from build123d import *

# Parameters (mm, degrees)
SKETCH1_W            = 133
SKETCH1_H            = 133
BOSS_EXTRUDE2_DEPTH  = 136
SKETCH2_W            = 133
SKETCH2_H            = 118
CUT_EXTRUDE1_DEPTH   = 136
BOSS_EXTRUDE3_DEPTH  = 10.5
SKETCH5_W            = 21
SKETCH5_H            = 3
BOSS_EXTRUDE4_DEPTH  = 23.5
SKETCH6_W            = 42
SKETCH6_H            = 17.2
CUT_EXTRUDE2_DEPTH   = 3
BOSS_EXTRUDE5_DEPTH  = 10.5
SKETCH8_W            = 21
SKETCH8_H            = 3
BOSS_EXTRUDE6_DEPTH  = 23.5
SKETCH9_W            = 42
SKETCH9_H            = 17.2
CUT_EXTRUDE3_DEPTH   = 3
SKETCH10_W           = 19.261488562
SKETCH10_H           = 133
BOSS_EXTRUDE7_DEPTH  = 5
SKETCH11_W           = 18.43727499
SKETCH11_H           = 133
BOSS_EXTRUDE8_DEPTH  = 5
SKETCH12_W           = 18.849381776
SKETCH12_H           = 146
BOSS_EXTRUDE9_DEPTH  = 12
SKETCH14_W           = 18.849381776
SKETCH14_H           = 146
BOSS_EXTRUDE10_DEPTH = 12
SKETCH17_R           = 1
CUT_EXTRUDE4_DEPTH   = 222.251553667
SKETCH18_W           = 133
SKETCH18_H           = 136
CUT_EXTRUDE5_DEPTH   = 170
SKETCH20_R           = 2.5
CUT_EXTRUDE6_DEPTH   = 10
SKETCH22_R           = 2.5
CUT_EXTRUDE8_DEPTH   = 170
SKETCH24_R           = 2.5
CUT_EXTRUDE9_DEPTH   = 170
SKETCH26_R           = 2.474722671
CUT_EXTRUDE10_DEPTH  = 177
SKETCH27_R           = 2.5
CUT_EXTRUDE11_DEPTH  = 177
SKETCH29_R           = 2.5
CUT_EXTRUDE12_DEPTH  = 177
SKETCH31_R           = 4
CUT_EXTRUDE13_DEPTH  = 173


with BuildPart() as part:
    # Sketch1 → Boss-Extrude2 (new body)
    with BuildSketch(Plane(origin=(0, 0, 0), x_dir=(1, 0, 0), z_dir=(0, 1, 0))):
        Rectangle(SKETCH1_W, SKETCH1_H)
    extrude(amount=BOSS_EXTRUDE2_DEPTH)

    # Sketch2 → Cut-Extrude1 (cut)
    with BuildSketch(Plane.XY.offset(66.5)):
        with Locations((0, 68)):
            Rectangle(SKETCH2_W, SKETCH2_H)
    extrude(amount=-CUT_EXTRUDE1_DEPTH, mode=Mode.SUBTRACT)


with BuildPart() as cut_extrude1_piece_1:
    # of the separate pieces the step leaves, piece 1, a body of its own (cut_extrude1_pieces)
    add(part.part.solids().sort_by_distance((-66.5, 0, 66.5))[0])

    # Sketch4 → Boss-Extrude3 (add)
    with BuildSketch(Plane(origin=(0, 9, 0), x_dir=(1, 0, 0), z_dir=(0, 1, 0))):
        Polygon((22.75, -22.75), (43.75, -22.75), (46.25, -22.75), (46.25, -20.25), (20.25, -20.25), (20.25, -46.25), (46.25, -46.25), (46.25, -43.75), (43.75, -43.75), (22.75, -43.75), align=None)
        Polygon((22.75, 43.75), (43.75, 43.75), (46.25, 43.75), (46.25, 46.25), (20.25, 46.25), (20.25, 20.25), (46.25, 20.25), (46.25, 22.75), (43.75, 22.75), (22.75, 22.75), align=None)
    extrude(amount=BOSS_EXTRUDE3_DEPTH)

    # Sketch5 → Boss-Extrude4 (add)
    with BuildSketch(Plane(origin=(22.75, 0, 0), x_dir=(0, 0, -1), z_dir=(1, 0, 0))):
        with Locations((-33.25, 18)):
            Rectangle(SKETCH5_W, SKETCH5_H)
        with Locations((33.25, 18)):
            Rectangle(SKETCH5_W, SKETCH5_H)
    extrude(amount=BOSS_EXTRUDE4_DEPTH)

    # Sketch6 → Cut-Extrude2 (cut)
    with BuildSketch(Plane(origin=(0, 19.5, 0), x_dir=(1, 0, 0), z_dir=(0, 1, 0))):
        with Locations((46.25, -33.25)):
            Rectangle(SKETCH6_W, SKETCH6_H)
        with Locations((46.25, 33.25)):
            Rectangle(SKETCH6_W, SKETCH6_H)
    extrude(amount=-CUT_EXTRUDE2_DEPTH, mode=Mode.SUBTRACT)

    # Sketch10 → Boss-Extrude7 (add)
    with BuildSketch(Plane.XZ):
        Rectangle(SKETCH10_W, SKETCH10_H)
    extrude(amount=BOSS_EXTRUDE7_DEPTH)



with BuildPart() as cut_extrude1_piece_2:
    # of the separate pieces the step leaves, piece 2, a body of its own (cut_extrude1_pieces)
    add(part.part.solids().sort_by_distance((66.5, 127, 66.5))[0])

    # Sketch7 → Boss-Extrude5 (add)
    with BuildSketch(Plane.XZ.offset(-127)):
        Polygon((-43.75, 43.75), (-22.75, 43.75), (-22.75, 22.75), (-43.75, 22.75), (-46.25, 22.75), (-46.25, 20.25), (-20.25, 20.25), (-20.25, 46.25), (-46.25, 46.25), (-46.25, 43.75), align=None)
        Polygon((-43.75, -22.75), (-22.75, -22.75), (-22.75, -43.75), (-43.75, -43.75), (-46.25, -43.75), (-46.25, -46.25), (-20.25, -46.25), (-20.25, -20.25), (-46.25, -20.25), (-46.25, -22.75), align=None)
    extrude(amount=BOSS_EXTRUDE5_DEPTH)

    # Sketch8 → Boss-Extrude6 (add)
    with BuildSketch(Plane.ZY.offset(22.75)):
        with Locations((33.25, 118)):
            Rectangle(SKETCH8_W, SKETCH8_H)
        with Locations((-33.25, 118)):
            Rectangle(SKETCH8_W, SKETCH8_H)
    extrude(amount=BOSS_EXTRUDE6_DEPTH)

    # Sketch9 → Cut-Extrude3 (cut)
    with BuildSketch(Plane.XZ.offset(-116.5)):
        with Locations((-46.25, 33.25)):
            Rectangle(SKETCH9_W, SKETCH9_H)
        with Locations((-46.25, -33.25)):
            Rectangle(SKETCH9_W, SKETCH9_H)
    extrude(amount=-CUT_EXTRUDE3_DEPTH, mode=Mode.SUBTRACT)

    # Sketch11 → Boss-Extrude8 (add)
    with BuildSketch(Plane(origin=(0, 136, 0), x_dir=(1, 0, 0), z_dir=(0, 1, 0))):
        Rectangle(SKETCH11_W, SKETCH11_H)
    extrude(amount=BOSS_EXTRUDE8_DEPTH)


with BuildPart() as cut_extrude1_piece_1_1:
    add(cut_extrude1_piece_1.part)

    add(cut_extrude1_piece_2.part)  # Boss-Extrude9 merges Cut-Extrude1 piece 2
    # Sketch12 → Boss-Extrude9 (add)
    with BuildSketch(Plane(origin=(0, 0, -66.5), x_dir=(-1, 0, 0), z_dir=(0, 0, -1))):
        with Locations((-0.206053393, 68)):
            Rectangle(SKETCH12_W, SKETCH12_H)
    extrude(amount=BOSS_EXTRUDE9_DEPTH)

    # Sketch14 → Boss-Extrude10 (add)
    with BuildSketch(Plane.XY.offset(66.5)):
        with Locations((0.206053393, 68)):
            Rectangle(SKETCH14_W, SKETCH14_H)
    extrude(amount=BOSS_EXTRUDE10_DEPTH)

    # Sketch17 → Cut-Extrude4 (cut, through all)
    with BuildSketch(Plane.XY.offset(78.5)):
        with Locations((0.206053393, 68)):
            Circle(SKETCH17_R)
    extrude(amount=-CUT_EXTRUDE4_DEPTH, mode=Mode.SUBTRACT)

    # Sketch18 → Cut-Extrude5 (cut)
    with BuildSketch(Plane.ZY.offset(66.5)):
        with Locations((0, 68)):
            Rectangle(SKETCH18_W, SKETCH18_H)
    extrude(amount=-CUT_EXTRUDE5_DEPTH, mode=Mode.SUBTRACT)

    # Sketch20 → Cut-Extrude6 (cut)
    with BuildSketch(Plane(origin=(0, 0, 0), x_dir=(1, 0, 0), z_dir=(0, 1, 0))):
        with Locations(Location((0, 0, 0), (0, 0, 270))):
            Circle(SKETCH20_R)
    extrude(amount=-CUT_EXTRUDE6_DEPTH, mode=Mode.SUBTRACT)

    # Sketch22 → Cut-Extrude8 (cut)
    with BuildSketch(Plane(origin=(0, 0, 0), x_dir=(1, 0, 0), z_dir=(0, 1, 0))):
        with Locations(Location((0, 0, 0), (0, 0, 270))):
            Circle(SKETCH22_R)
    extrude(amount=CUT_EXTRUDE8_DEPTH, mode=Mode.SUBTRACT)

    # Sketch24 → Cut-Extrude9 (cut)
    with BuildSketch(Plane(origin=(0, 0, 0), x_dir=(1, 0, 0), z_dir=(0, 1, 0))):
        with Locations(Location((0, 59.159797643, 0), (0, 0, 270))):
            Circle(SKETCH24_R)
    extrude(amount=-CUT_EXTRUDE9_DEPTH, mode=Mode.SUBTRACT)

    # Sketch26 → Cut-Extrude10 (cut)
    with BuildSketch(Plane(origin=(0, 9, 0), x_dir=(1, 0, 0), z_dir=(0, 1, 0))):
        with Locations(Location((0, 59.159797643, 0), (0, 0, 90))):
            Circle(SKETCH26_R)
    extrude(amount=CUT_EXTRUDE10_DEPTH, mode=Mode.SUBTRACT)

    # Sketch27 → Cut-Extrude11 (cut)
    with BuildSketch(Plane(origin=(0, 0, 0), x_dir=(1, 0, 0), z_dir=(0, 1, 0))):
        with Locations(Location((0, -59.499471122, 0), (0, 0, 270))):
            Circle(SKETCH27_R)
    extrude(amount=-CUT_EXTRUDE11_DEPTH, mode=Mode.SUBTRACT)

    # Sketch29 → Cut-Extrude12 (cut)
    with BuildSketch(Plane.XZ.offset(5)):
        with Locations(Location((0, 59.499471122, 0), (0, 0, 90))):
            Circle(SKETCH29_R)
    extrude(amount=-CUT_EXTRUDE12_DEPTH, mode=Mode.SUBTRACT)

    # Sketch31 → Cut-Extrude13 (cut)
    with BuildSketch(Plane(origin=(0, 141, 0), x_dir=(1, 0, 0), z_dir=(0, 1, 0))):
        with Locations(Location((0, 0, 0), (0, 0, 270))):
            Circle(SKETCH31_R)
    extrude(amount=-CUT_EXTRUDE13_DEPTH, mode=Mode.SUBTRACT)


solid = cut_extrude1_piece_1_1.part
The listing builds one solid part. Answer for the finished solid, in the listing's coordinates (mm). A direction names the side the tool comes from. Coordinates: 2 decimals unless noted, no trailing zeros. Order: outer loops, then holes, each group sorted by start corner. A loop starts at its lowest first (then second) coordinate and runs counter-clockwise, first axis right, second up. Notation, with made-up numbers: (45, 12) -> (68, 12) arc R24 cw to (68, 33) -> close; hole circle Ø3 at (70.25, 22.25). An arc over 180 degrees is marked (long way). Answer in a Markdown table with one row per item. Add a question column.
Item 1: Which of the six approach directions +Z, -Z, +X, -X, +Y, -Y give full straight-line access (tool end or side, diameter ignored) to faces 5 (the face through (-4.4, -5, -1.1)), 6 (the face through (9.219, 138, 1)), 7 (the face through (-4.2, 136, -0.9))?
Item 2: Find section A-A (z = 0). Write down the section's boundary in (x, y).
Item 3: Determine the mould class of faces 1 (the face through (0, -2, 57)), 2 (the face through (9.631, -3, 0)), 3 (the face through (0.11, -2.465, -61.657)), 4 (the face through (-2, 69, 78.5)) for opening direction Z: +Z half, -Z half, draft (parallel to the pull), parting line (faces both ways), or undercut.
Item 4: Find section C-C (z = 32.5). Write down the section's boundary in (x, y).
Item 5: Find section B-B (y = 13). Write down the section's boundary in (x, z), then the cut area to 3 significant figures.
Item 6: Each of these flat-tipped pins is pushed along its axis until it touches: P1, Ø0.5, axis at x = -9.5, y = -2.5, coming from the -Z side; P2, Ø1.5, axis at y = 139, z = 6, coming from the +X side. Where does it stop, or does it pass through?
Item 7: Find the intervals of material crossed by L1, parallel to Y at x = 4, z = -59.5; L2, parallel to X at y = -3.9, z = 0; L3, parallel to Z at x = 8.25, y = 18, in increasing order. Write a range as from..to.
Result set:
| question | item | result |
|---|---|---|
| 1 | face 5 | +Z, -Z, +X, -X, -Y |
| 1 | face 6 | +X, +Y |
| 1 | face 7 | +X, -X |
| 2 | outline | (-9.63, -5) -> (-4, -5) -> (-4, 0) -> (-9.63, 0) -> close; (-9.22, 136) -> (-4, 136) -> (-4, 141) -> (-9.22, 141) -> close; (4, -5) -> (9.63, -5) -> (9.63, 0) -> (4, 0) -> close; (4, 136) -> (9.22, 136) -> (9.22, 141) -> (4, 141) -> close |
| 3 | face 1 | undercut |
| 3 | face 2 | draft |
| 3 | face 3 | undercut |
| 3 | face 4 | +Z half |
| 4 | outline | (-9.63, -5) -> (9.63, -5) -> (9.63, 0) -> (-9.63, 0) -> close; (-9.22, 136) -> (9.22, 136) -> (9.22, 141) -> (-9.22, 141) -> close |
| 5 | outline | (-9.22, -78.5) -> (9.63, -78.5) -> (9.63, -66.5) -> (-9.22, -66.5) -> close; (-9.22, 66.5) -> (9.63, 66.5) -> (9.63, 78.5) -> (-9.22, 78.5) -> close |
| 5 | area | 452 mm² |
| 6 | P1 | stops at z = -66.5 |
| 6 | P2 | stops at x = 9.22 |
| 7 | L1 | y = -5..0, 136..141 |
| 7 | L2 | x = -9.63..-4, 4..9.63 |
| 7 | L3 | z = -78.5..-66.5, 66.5..78.5 |
